from build123d import *

# Parameters (mm, degrees)
F0_W     = 367.04778
F0_H     = 31.496
F1_DEPTH = 457.2
F2_W     = 355.6
F2_H     = 367.04778
F3_DEPTH = 3.302
F4_W     = 355.6
F4_H     = 34.798
F5_DEPTH = 3.302


with BuildPart() as f1:
    # F0 (on Right) → F1 (new body)
    with BuildSketch(Plane.YZ):
        Rectangle(F0_W, F0_H)
    extrude(amount=F1_DEPTH)

    # F2 (on face) → F3 (join)
    with BuildSketch(Plane.XY.offset(15.748)):
        with Locations((228.6, 0)):
            Rectangle(F2_W, F2_H)
    extrude(amount=F3_DEPTH)

    # F4 (on face) → F5 (join)
    with BuildSketch(Plane.XZ.offset(183.52389)):
        with Locations((228.6, 1.651)):
            Rectangle(F4_W, F4_H)
    extrude(amount=F5_DEPTH)


solid = f1.part
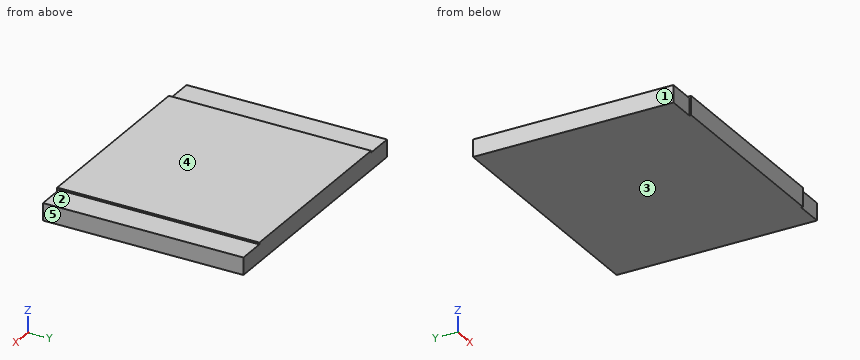
Can you work these out from the model? Positions are in its coordinate system, mm. Face numbers are marked on the shaded views. A direction names the side the tool comes from. Round coordinates to 2 decimals unless told otherwise and drop trailing zeros. Order: outer loops, then holes, each group sorted by start corner. A loop starts at its lowest first (then second) coordinate and runs counter-clockwise, first axis right, second up. Notation, with made-up numbers: M -20,39 L 29,39 A26 cw 29,53 Z; hole C 17.5,9.5 d9. An arc over 180 degrees is marked long. Use a Markdown table: item, result.
1) If I drill on line 1 along X through (y, z) = (-27, 18); line 2 along Y through (x, z) = (24, -13); line 3 along Z through (x, y) = (22, 16), over which ranges is the centre line in solid material (lowest first)?
Geometry says:
| item | result |
|---|---|
| line 1 | x = 50.8 to 406.4 |
| line 2 | y = -183.52 to 183.52 |
| line 3 | z = -15.75 to 15.75 |
2) If we mould it in two halves opening along Z, with no side actions, what happens to the marked faces 3, 4 and 5? For each: +Z half, -Z half, draft (parallel to the pull), parting line (faces both ways), or undercut.
Geometry says:
| item | result |
|---|---|
| face 3 | -Z half |
| face 4 | +Z half |
| face 5 | draft |
3) Imagine slicing it at A-A (y = 150.5). List the corners of the cut face in (x, z) for me, then the cut area to 3 significant figures.
Geometry says:
| item | result |
|---|---|
| outline | M 0,-15.75 L 457.2,-15.75 L 457.2,15.75 L 406.4,15.75 L 406.4,19.05 L 50.8,19.05 L 50.8,15.75 L 0,15.75 Z |
| area | 15,600 mm² |
4) On a 3-axis mill with a long thin cutter (end or side, diameter ignored), from which of +Z, -Z, +X, -X, +Y, -Y can I reach the whole of each face in a straight line? I mean the marked faces 1 and 2. Say none if no direction works.
Geometry says:
| item | result |
|---|---|
| face 1 | +Z, -Z, -X, +Y, -Y |
| face 2 | +Z, +X, +Y, -Y |
5) I'm going to push flat-ended pins straight in: P1, Ø12, axis at y = -97.5, z = 11, coming from the -X side; P2, Ø9.5, axis at x = 36.5, z = 5, coming from the -Y side. Where does each tip first touch, or does it pass through?
Geometry says:
| item | result |
|---|---|
| P1 | stops at x = 0 |
| P2 | stops at y = -183.52 |
